from build123d import *

# Parameters (mm, degrees)
SCHIZZO2_R                   = 145
SCHIZZO2_R_2                 = 105
ESTRUSIONE_ESTRUSIONE2_START = -50
SCHIZZO5_W                   = 360
SCHIZZO5_H                   = 357.468314384
SCHIZZO5_R                   = 145
ESTRUSIONE_ESTRUSIONE2_DEPTH = 50
RACCORDO2_R                  = 20
SCHIZZO11_R                  = 145
ESTRUSIONE_ESTRUSIONE3_DEPTH = 50
SCHIZZO12_R                  = 30
TAGLIO_ESTRUSIONE1_DEPTH     = 10
TAGLIO_ESTRUSIONE2_REACH     = 741.709
SCHIZZO13_R                  = 15
RIPETIZIONECIRCOLARE1_COUNT  = 4
SCHIZZO14_R                  = 30
TAGLIO_ESTRUSIONE3_DEPTH     = 10
TAGLIO_ESTRUSIONE4_REACH     = 856.322
SCHIZZO16_R                  = 15
RIPETIZIONECIRCOLARE2_COUNT  = 4
SMUSSO1_SIZE                 = 10


with BuildPart() as part:
    # Sweep-Sottile1: sweep along a path in Schizzo1
    with BuildLine(Plane.XY) as sweep_sottile1_path:
        Line((0, 0), (-150, 0))
        ThreePointArc((-150, 0), (-333.847763109, 76.152236891), (-410, 260))
        Line((-410, 260), (-410, 422.338378292))
    # Schizzo2 → Sweep-Sottile1 (sweep)
    with BuildSketch(Plane(origin=(0, 0, 0), x_dir=(0, 0, -1), z_dir=(1, 0, 0))):
        Circle(SCHIZZO2_R)
        Circle(SCHIZZO2_R_2, mode=Mode.SUBTRACT)
    sweep(path=sweep_sottile1_path.line)

    # Schizzo5 → Estrusione-Estrusione2 (add)
    with BuildSketch(Plane(origin=(0, 0, 0), x_dir=(0, 0, -1), z_dir=(1, 0, 0)).offset(ESTRUSIONE_ESTRUSIONE2_START)):
        Rectangle(SCHIZZO5_W, SCHIZZO5_H)
        with Locations(Location((0, 0, 0), (0, 0, 270))):
            Circle(SCHIZZO5_R, mode=Mode.SUBTRACT)
    extrude(amount=ESTRUSIONE_ESTRUSIONE2_DEPTH)

    # Raccordo2
    raccordo2_edges = [part.edges().sort_by_distance(p)[0] for p in [
        (-25, -178.734157192, -180),
        (-25, -178.734157192, 180),
        (-25, 178.734157192, 180),
        (-25, 178.734157192, -180),
    ]]
    fillet(raccordo2_edges, radius=RACCORDO2_R)

    # Schizzo11 → Estrusione-Estrusione3 (add)
    with BuildSketch(Plane(origin=(0, 422.338378292, 0), x_dir=(1, 0, 0), z_dir=(0, 1, 0))):
        with BuildLine():
            ThreePointArc((-250, 180), (-235.857864376, 174.142135624), (-230, 160))
            Line((-230, 160), (-230, -160))
            ThreePointArc((-230, -160), (-235.857864376, -174.142135624), (-250, -180))
            Line((-250, -180), (-570, -180))
            ThreePointArc((-570, -180), (-584.142135624, -174.142135624), (-590, -160))
            Line((-590, -160), (-590, 160))
            ThreePointArc((-590, 160), (-584.142135624, 174.142135624), (-570, 180))
            Line((-570, 180), (-250, 180))
        make_face()
        with Locations(Location((-410, 0, 0), (0, 0, 270))):
            Circle(SCHIZZO11_R, mode=Mode.SUBTRACT)
    extrude(amount=-ESTRUSIONE_ESTRUSIONE3_DEPTH)

    # Schizzo12 → Taglio-Estrusione1 (cut)
    with BuildSketch(Plane(origin=(0, 0, 0), x_dir=(0, 0, -1), z_dir=(1, 0, 0))):
        with Locations((-130, 130)):
            Circle(SCHIZZO12_R)
    taglio_estrusione1 = extrude(amount=-TAGLIO_ESTRUSIONE1_DEPTH, mode=Mode.SUBTRACT)

    # Schizzo13 → Taglio-Estrusione2 (cut, up to next)
    with BuildSketch(Plane(origin=(-10, 0, 0), x_dir=(0, 0, -1), z_dir=(1, 0, 0)), mode=Mode.PRIVATE) as taglio_estrusione2_sk1:
        with Locations((-130, 130)):
            Circle(SCHIZZO13_R)
    taglio_estrusione2_tool1 = extrude(taglio_estrusione2_sk1.sketch, amount=-TAGLIO_ESTRUSIONE2_REACH, mode=Mode.PRIVATE) & part.part
    taglio_estrusione2 = taglio_estrusione2_tool1.solids().sort_by_distance((-10, 130, 130))[0]
    add(taglio_estrusione2, mode=Mode.SUBTRACT)

    # RipetizioneCircolare1: Taglio-Estrusione1, Taglio-Estrusione2 ×4 about axis
    ripetizionecircolare1_axis = Axis((0, 0, 0), (1, 0, 0))
    add([taglio_estrusione1.rotate(ripetizionecircolare1_axis, i * 360 / RIPETIZIONECIRCOLARE1_COUNT) for i in range(1, RIPETIZIONECIRCOLARE1_COUNT)], mode=Mode.SUBTRACT)
    add([taglio_estrusione2.rotate(ripetizionecircolare1_axis, i * 360 / RIPETIZIONECIRCOLARE1_COUNT) for i in range(1, RIPETIZIONECIRCOLARE1_COUNT)], mode=Mode.SUBTRACT)

    # Schizzo14 → Taglio-Estrusione3 (cut)
    with BuildSketch(Plane(origin=(0, 422.338378292, 0), x_dir=(1, 0, 0), z_dir=(0, 1, 0))):
        with Locations(Location((-540, 130, 0), (0, 0, 270))):
            Circle(SCHIZZO14_R)
    taglio_estrusione3 = extrude(amount=-TAGLIO_ESTRUSIONE3_DEPTH, mode=Mode.SUBTRACT)

    # Schizzo16 → Taglio-Estrusione4 (cut, up to next)
    with BuildSketch(Plane(origin=(0, 412.338378292, 0), x_dir=(1, 0, 0), z_dir=(0, 1, 0)), mode=Mode.PRIVATE) as taglio_estrusione4_sk1:
        with Locations(Location((-540, 130, 0), (0, 0, 270))):
            Circle(SCHIZZO16_R)
    taglio_estrusione4_tool1 = extrude(taglio_estrusione4_sk1.sketch, amount=-TAGLIO_ESTRUSIONE4_REACH, mode=Mode.PRIVATE) & part.part
    taglio_estrusione4 = taglio_estrusione4_tool1.solids().sort_by_distance((-540, 412.338378, -130))[0]
    add(taglio_estrusione4, mode=Mode.SUBTRACT)

    # RipetizioneCircolare2: Taglio-Estrusione3, Taglio-Estrusione4 ×4 about axis
    ripetizionecircolare2_axis = Axis((-410, 0, 0), (0, 1, 0))
    add([taglio_estrusione3.rotate(ripetizionecircolare2_axis, i * 360 / RIPETIZIONECIRCOLARE2_COUNT) for i in range(1, RIPETIZIONECIRCOLARE2_COUNT)], mode=Mode.SUBTRACT)
    add([taglio_estrusione4.rotate(ripetizionecircolare2_axis, i * 360 / RIPETIZIONECIRCOLARE2_COUNT) for i in range(1, RIPETIZIONECIRCOLARE2_COUNT)], mode=Mode.SUBTRACT)

    # Smusso1
    smusso1_edges = [part.edges().sort_by_distance(p)[0] for p in [
        (0, 0, 105),
        (-410, 422.338378292, 105),
    ]]
    chamfer(smusso1_edges, length=SMUSSO1_SIZE)


solid = part.part
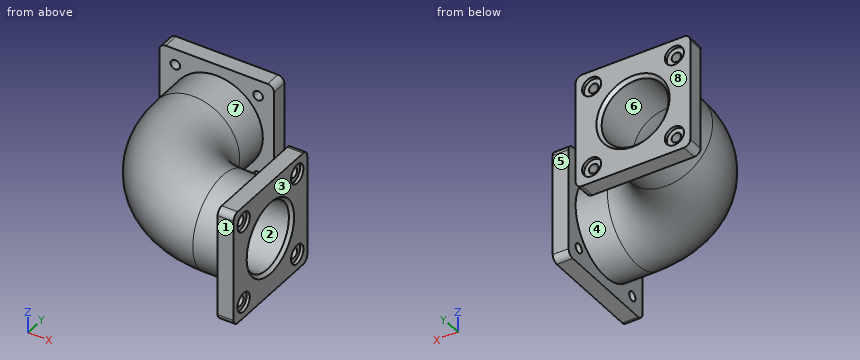
Model file for the job. Use its own axes, mm. Face numbers are marked on the shaded views. A direction names the side the tool comes from. Give positions to 0.01 mm unless a question says otherwise; leave off trailing zeros. Loops run counter-clockwise (first coordinate to the right, second up) from the corner with the lowest first, then second, coordinate; pieces in that order, holes last.
Item 1: Drill centre lines: line 1 along X through (y, z) = (417, 130); line 2 along Z through (x, y) = (-6.5, -130); line 3 along X through (y, z) = (171, -2). Where is each one in solid material? Low to high.
Check values:
line 1: x = -590 to -570, -510 to -310, -250 to -230
line 2: z = -180 to -160, -100 to 100, 160 to 180
line 3: x = -545.09 to -503.96, -276.92 to -222.85, -50 to 0
Item 2: Mould opens along Z. For the marked faces 6, 7 and 8 say: +Z half, -Z half, draft (parallel to the pull), parting line (faces both ways), or undercut.
Check values:
face 6: undercut
face 7: parting line
face 8: draft
Item 3: Slice it at D-D (x = -280). Give the number of separate pieces and of enclosed holes in the cut face, plus the area to 3 significant figures.
Check values:
separate pieces: 3
enclosed holes: 1
area: 73,200 mm2
Item 4: Slice it at A-A (z = 0). Write the cut outline in (x, y).
Check values:
outline: (-590, 372.34) - (-555, 372.34) - (-555, 260) arc R405 ccw to (-150, -145) - (-50, -145) - (-50, -178.73) - (0, -178.73) - (0, -115) - (-10, -105) - (-150, -105) arc R365 cw to (-515, 260) - (-515, 412.34) - (-525, 422.34) - (-590, 422.34) - close; (-305, 260) arc R155 ccw to (-150, 105) - (-10, 105) - (0, 115) - (0, 178.73) - (-50, 178.73) - (-50, 145) - (-150, 145) arc R115 cw to (-265, 260) - (-265, 372.34) - (-230, 372.34) - (-230, 422.34) - (-295, 422.34) - (-305, 412.34) - close
Item 5: Which spindle directions (+Z, -Z, +X, -X, +Y, -Y) get a long thin tool onto all of the face, cutting with end or side? Do the marked faces 1, 2, 3, 4 and 5. Say none if no direction does.
Check values:
face 1: +Z, -Z, +X, -X, -Y
face 2: +X
face 3: +Z, -Z, +X, +Y, -Y
face 4: none
face 5: +Z, -Z, +X, +Y
Item 6: Drop flat-ended pins along their axis: P1, Ø18, axis at x = -540, z = 130, coming from the +Y side; P2, Ø3, axis at x = -326.5, z = -61.5, coming from the -Y side; P3, Ø25, axis at x = -12.5, z = 31.5, coming from the +Y side; P4, Ø1.5, axis at x = -362.5, y = -33, coming from the +Z side. Give the stop position or say it passes through.
Check values:
P1: passes through
P2: stops at y = -90.33
P3: stops at y = 178.73
P4: stops at z = 103.85
Item 7: Slice it at C-C (x = -81). Write the cut outline in (y, z), plus the area to 3 significant figures.
Check values:
outline: circle Ø290 at (0, 0); hole circle Ø210 at (0, 0)
area: 31,400 mm2
Item 8: Slice it at B-B (y = 385.5). Write the cut outline in (x, z), plus the area to 3 significant figures.
Check values:
outline: (-590, -160) arc R20 ccw to (-570, -180) - (-250, -180) arc R20 ccw to (-230, -160) - (-230, 160) arc R20 ccw to (-250, 180) - (-570, 180) arc R20 ccw to (-590, 160) - close; hole circle Ø30 at (-540, -130); hole circle Ø30 at (-540, 130); hole circle Ø210 at (-410, 0); hole circle Ø30 at (-280, -130); hole circle Ø30 at (-280, 130)
area: 91,800 mm2
